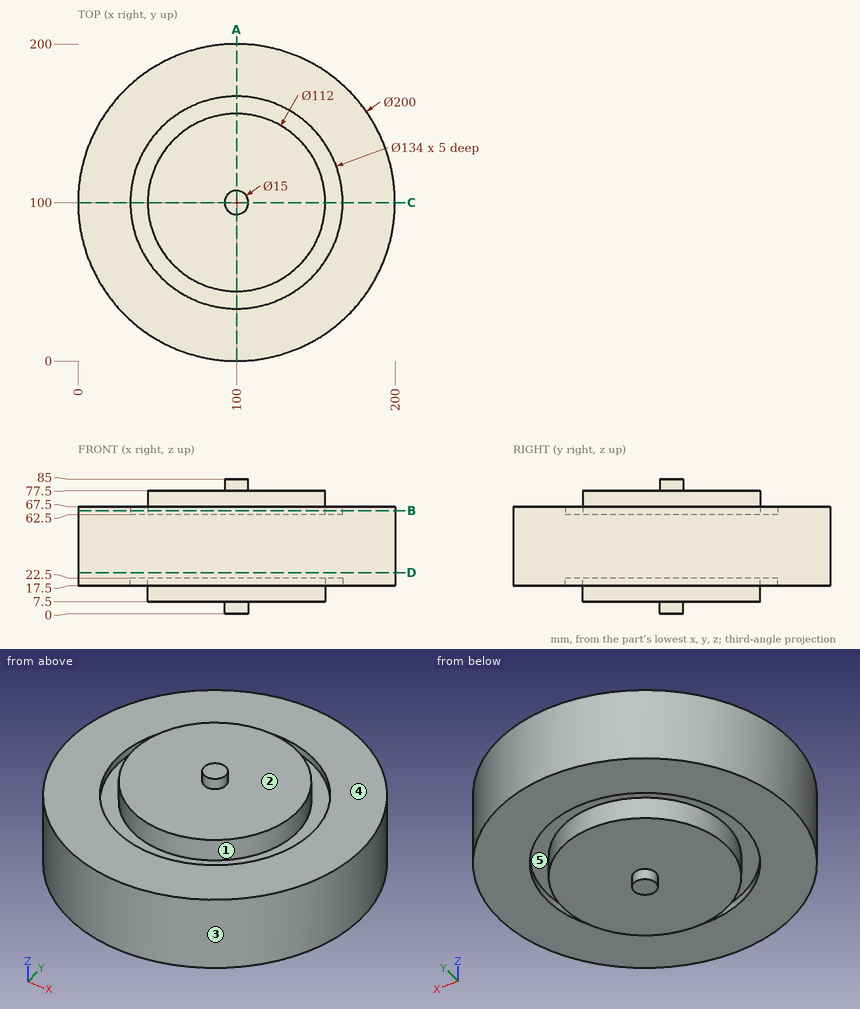
For this review, use the dimensioned drawing (mm, ordinates from the lowest corner) and the shaded views. A direction names the side the tool comes from. Round coordinates to 2 decimals unless told otherwise and drop trailing zeros. Loops run counter-clockwise (first coordinate to the right, second up) from the corner with the lowest first, then second, coordinate; pieces in that order, holes last. Notation, with made-up numbers: (56, -9.75) -> (76, -9.75) arc R24 cw to (76, 25.25) -> close; hole circle Ø4 at (-31.75, 86). An arc over 180 degrees is marked (long way). Write item = value, one per line. Start each with the question number.
Item 1: Mouldability with a two-part tool opening along Y and no side actions: class the marked faces 1, 2 and 3 as released by +Y, released by -Y, zero draft, split by the parting line, or undercut.
Item 2: Take a section at A-A on x = 100. Give the boundary of the cut face in (y, z).
Item 3: Take a section at B-B on z = 65. Give the boundary of the cut face in (x, y), plus the area to 3 significant figures.
Item 4: To check wall thickness, follow L1, parallel to Y at x = 100, z = 18; L2, parallel to Z at x = 42.5, y = 120.5; L3, parallel to Z at x = 39.5, y = 167.5. State the ranges of each line that lie inside material, in increasing order.
Item 5: For the marked faces 4 and 5, list the 3-axis set-ups (+Z, -Z, +X, -X, +Y, -Y) from which the entire face can be reached by the end or side of a thin tool; tool diameter is ignored.
Item 6: Take a section at D-D on z = 26. Give the boundary of the cut face in (x, y).
Item 7: Insertion check: pin 1 (1.5 mm diameter, centred on x = 104, y = 46.5, fed in from -Z); pin 2 (4 mm diameter, centred on x = 120.5, y = 40, fed in from -Z); pin 3 (4 mm diameter, centred on y = 114.5, z = 70.5, fed in from +X). Each pin has a flat end and moves straight along its axis. Give the tip position at first contact, or say it passes through.
Result:
q1.face_1 = undercut
q1.face_2 = zero draft
q1.face_3 = split by the parting line
q2.outline = (0, 17.5) -> (33, 17.5) -> (33, 22.5) -> (44, 22.5) -> (44, 7.5) -> (92.5, 7.5) -> (92.5, 0) -> (107.5, 0) -> (107.5, 7.5) -> (156, 7.5) -> (156, 22.5) -> (167, 22.5) -> (167, 17.5) -> (200, 17.5) -> (200, 67.5) -> (167, 67.5) -> (167, 62.5) -> (156, 62.5) -> (156, 77.5) -> (107.5, 77.5) -> (107.5, 85) -> (92.5, 85) -> (92.5, 77.5) -> (44, 77.5) -> (44, 62.5) -> (33, 62.5) -> (33, 67.5) -> (0, 67.5) -> close
q3.outline = circle Ø200 at (100, 100); circle Ø112 at (100, 100); hole circle Ø134 at (100, 100)
q3.area = 27,200 mm²
q4.L1 = 0 to 33, 44 to 156, 167 to 200
q4.L2 = 22.5 to 62.5
q4.L3 = 17.5 to 67.5
q5.face_4 = +Z
q5.face_5 = -Z
q6.outline = circle Ø200 at (100, 100)
q7.pin_1 = 7.5
q7.pin_2 = 22.5
q7.pin_3 = 154.59
